Autodesk Inventor part; units mm, degrees
ref_plane "YZ Plane" through (0, 0, 0) normal (1, 0, 0) x (0, 1, 0)
ref_plane "XZ Plane" through (0, 0, 0) normal (0, 1, 0) x (-1, 0, 0)
ref_plane "XY Plane" through (0, 0, 0) normal (0, 0, 1) x (1, 0, 0)
sketch "Sketch1" plane through (0, 0, 0) normal (0, 0, 1) x (1, 0, 0)
  line L0 (0, 0) -> (12, 0)
  line L1 (12, 0) -> (12, 25)
  line L2 (12, 25) -> (0, 25)
  line L3 (0, 25) -> (0, 0)
  dimension "d0" = 12
  dimension "d1" = 25
extrude "Extrusion1" add sketch "Sketch1" along normal blind 10
sketch "Sketch2" plane through (0, 25, 0) normal (0, 1, 0) x (1, 0, 0)
  line L0 (12, 0) -> (0, 0) construction
  line L1 (0, 0) -> (0, -10) construction
  line L2 (12, -10) -> (0, -10) construction
  line L3 (12, 0) -> (12, -10) construction
  circle A0 centre (6, -5) radius 1.5
  point P0 (12, -5)
  point P1 (6, -10)
  dimension "d4" = 3
extrude "Extrusion2" add sketch "Sketch2" along normal blind 6
sketch "Sketch3" plane through (6, 31, 5) normal (0, 1, 0) x (1, 0, 0)
  circle A0 centre (0, 0) radius 1.5 construction
  circle A1 centre (0, 0) radius 40
  point P0 (-6, 5)
  dimension "d7" = 80
extrude "Extrusion3" add sketch "Sketch3" along normal blind 10
properties part number "Wheel and Motor"
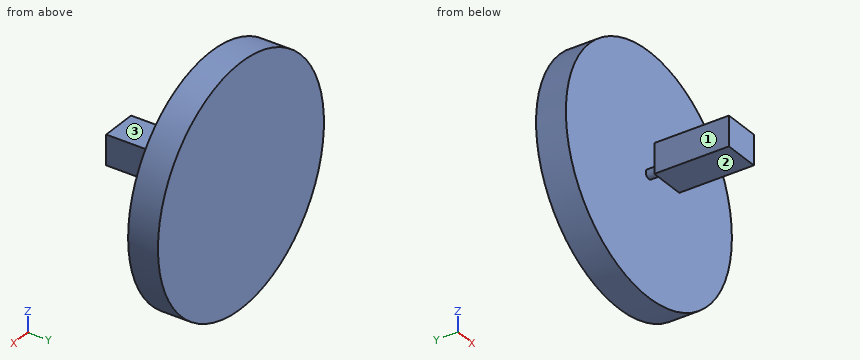
CAD build for the part. Positions are in the model's coordinates, mm. Face numbers are marked on the shaded views. A direction names the side the tool comes from. Coordinates: 2 decimals unless noted, no trailing zeros. Order: outer loops, then holes, each group sorted by start corner. A loop starts at its lowest first (then second) coordinate and runs counter-clockwise, first axis right, second up.
(1) Drill centre lines: L1, parallel to Y at x = -6, z = 41.5; L2, parallel to X at y = 7.5, z = 4; L3, parallel to Z at x = 3.5, y = 3. Where is each one in solid material? Low to high.
Solution:
L1: y = 31 to 41
L2: x = 0 to 12
L3: z = 0 to 10
(2) Saw through at D-D, the plane y = 3. Write the cut outline in (x, z).
Solution:
outline: (0, 0) - (12, 0) - (12, 10) - (0, 10) - close
(3) Pin check, flat tips, straight feed: pin 1 Ø9.5 at (x, y) = (6, 10) entering from -Z; pin 2 Ø10 at (x, y) = (-24.5, 28.5) entering from -Z; pin 3 Ø5 at (y, z) = (13.5, 4.5) entering from -X. Stop position of each tip, or through.
Solution:
pin 1: stops at z = 0
pin 2: stops at z = -25.25
pin 3: stops at x = 0
(4) Saw through at A-A, the plane x = 11. Write the cut outline in (y, z), and give its area (3 significant figures).
Solution:
outline: (0, 0) - (25, 0) - (25, 10) - (0, 10) - close; (31, -34.69) - (41, -34.69) - (41, 44.69) - (31, 44.69) - close
area: 1,040 mm2
(5) Saw through at B-B, the plane z = 5. Write the cut outline in (x, y).
Solution:
outline: (-34, 31) - (4.5, 31) - (4.5, 25) - (0, 25) - (0, 0) - (12, 0) - (12, 25) - (7.5, 25) - (7.5, 31) - (46, 31) - (46, 41) - (-34, 41) - close
(6) Which spindle directions (+Z, -Z, +X, -X, +Y, -Y) get a long thin tool onto all of the face, cutting with end or side? Do the marked faces 1, 2 and 3. Say none if no direction does.
Solution:
face 1: +Z, -Z, -X, -Y
face 2: -Z, +X, -X, -Y
face 3: +Z, +X, -X, -Y
(7) Saw through at C-C, the plane y = 37. Write the cut outline in (x, z).
Solution:
outline: circle Ø80 at (6, 5)
